Design review of the part built by this model. Coordinates are the model's own, in mm. A direction names the side the tool comes from. Give positions to 0.01 mm unless a question says otherwise; leave off trailing zeros. Order: outer loops, then holes, each group sorted by start corner. A loop starts at its lowest first (then second) coordinate and runs counter-clockwise, first axis right, second up. Notation, with made-up numbers: M 9.25,81 L 47.25,81 A14 ccw 47.25,91 Z; hole C 68,26 d2. An arc over 180 degrees is marked long. Put each result on its own line as item: value. Start each with the question number.
Autodesk Inventor part; units mm, degrees
ref_plane "YZ Plane" through (0, 0, 0) normal (1, 0, 0) x (0, 1, 0)
ref_plane "XZ Plane" through (0, 0, 0) normal (0, 1, 0) x (-1, 0, 0)
ref_plane "XY Plane" through (0, 0, 0) normal (0, 0, 1) x (1, 0, 0)
sketch "Sketch1" plane through (0, 0, 0) normal (0, 0, 1) x (1, 0, 0)
  line L0 (0, 68.5) -> (0, 6.5)
  line L1 (68, 68.5) -> (78, 58.5)
  line L2 (78, 58.5) -> (78, 16.5)
  line L3 (78, 16.5) -> (68, 6.5)
  line L4 (68, 0) -> (68, 6.5)
  line L5 (68, 68.5) -> (68, 75)
  circle A0 centre (71, 57.5) radius 2.75
  circle A1 centre (71, 17.5) radius 2.75
  line L6 (25, 67.5) -> (34, 67.5)
  line L7 (35, 66.5) -> (35, 43.5)
  line L8 (34, 42.5) -> (25, 42.5)
  line L9 (24, 43.5) -> (24, 66.5)
  line L10 (25, 32.5) -> (34, 32.5)
  line L11 (35, 31.5) -> (35, 8.5)
  line L12 (34, 7.5) -> (25, 7.5)
  line L13 (24, 8.5) -> (24, 31.5)
  arc A2 (25, 67.5) -> (24, 66.5) centre (25, 66.5) ccw
  arc A3 (35, 66.5) -> (34, 67.5) centre (34, 66.5) ccw
  arc A4 (34, 42.5) -> (35, 43.5) centre (34, 43.5) ccw
  arc A5 (24, 43.5) -> (25, 42.5) centre (25, 43.5) ccw
  arc A6 (25, 32.5) -> (24, 31.5) centre (25, 31.5) ccw
  arc A7 (24, 8.5) -> (25, 7.5) centre (25, 8.5) ccw
  arc A8 (34, 7.5) -> (35, 8.5) centre (34, 8.5) ccw
  arc A9 (35, 31.5) -> (34, 32.5) centre (34, 31.5) ccw
  line L14 (29.5, 67.5) -> (29.5, 7.5) construction
  circle A10 centre (6, 64.5) radius 5 construction
  circle A11 centre (6, 64.5) radius 2.75
  circle A12 centre (6, 10.5) radius 5 construction
  circle A13 centre (6, 10.5) radius 2.75
  line L15 (0, 64.5) -> (72, 64.5) construction
  line L16 (0, 10.5) -> (72, 10.5) construction
  line L17 (0, 6.5) -> (16, 6.5)
  line L18 (16, 6.5) -> (16, 0)
  line L19 (0, 68.5) -> (16, 68.5)
  line L20 (16, 68.5) -> (16, 75)
  line L21 (46, 75) -> (46, 68.5)
  line L22 (46, 68.5) -> (64, 68.5)
  line L23 (64, 68.5) -> (64, 75)
  line L24 (46, 0) -> (46, 6.5)
  line L25 (46, 6.5) -> (64, 6.5)
  line L26 (64, 6.5) -> (64, 0)
  line L27 (68, 75) -> (64, 75)
  line L28 (46, 75) -> (16, 75)
  line L29 (16, 0) -> (46, 0)
  line L30 (64, 0) -> (68, 0)
  line L31 (8, 60.5) -> (16, 60.5)
  line L32 (16, 60.5) -> (16, 54)
  line L33 (16, 54) -> (8, 54)
  line L34 (8, 54) -> (8, 60.5)
  line L35 (8, 21) -> (16, 21)
  line L36 (16, 21) -> (16, 14.5)
  line L37 (16, 14.5) -> (8, 14.5)
  line L38 (8, 14.5) -> (8, 21)
  line L39 (54, 21) -> (62, 21)
  line L40 (62, 21) -> (62, 14.5)
  line L41 (62, 14.5) -> (54, 14.5)
  line L42 (54, 14.5) -> (54, 21)
  line L43 (54, 60.5) -> (62, 60.5)
  line L44 (62, 60.5) -> (62, 54)
  line L45 (62, 54) -> (54, 54)
  line L46 (54, 54) -> (54, 60.5)
  circle A14 centre (14, 37.5) radius 5 construction
  circle A15 centre (46, 37.5) radius 5 construction
  circle A16 centre (46, 37.5) radius 2.75
  circle A17 centre (14, 37.5) radius 2.75
  point P0 (0, 0)
  point P1 (29.5, 37.5)
  point P2 (0, 37.5)
  dimension "d1" = 45
  dimension "d2" = 10
  dimension "d11" = 5.5
  dimension "d12" = 5.5
  dimension "d13" = 7
  dimension "d14" = 11
  dimension "d15" = 11
  dimension "d18" = 1
  dimension "d19" = 11
  dimension "d20" = 25
  dimension "d21" = 25
  dimension "d24" = 38.5
  dimension "d25" = 5.5
  dimension "d26" = 5.5
  dimension "d27" = 10
  dimension "d28" = 10
  dimension "d32" = 6
  dimension "d34" = 68
  dimension "d35" = 6.5
  dimension "d36" = 6.5
  dimension "d37" = 4
  dimension "d38" = 4
  dimension "d40" = 1
  dimension "d41" = 30
  dimension "d42" = 18
  dimension "d43" = 4
  dimension "d44" = 4
  dimension "d45" = 6.5
  dimension "d46" = 6.5
  dimension "d47" = 8
  dimension "d48" = 8
  dimension "d49" = 4
  dimension "d50" = 4
  dimension "d51" = 8
  dimension "d52" = 6
  dimension "d53" = 10
  dimension "d54" = 5.5
  dimension "d55" = 10
  dimension "d56" = 5.5
  dimension "d57" = 14
  dimension "d58" = 32
  dimension "d67" = 54
extrude "Extrusion1" add sketch "Sketch1" along normal blind 6.5
sketch "Sketch2" plane through (0, 0, 6.5) normal (0, 0, 1) x (1, 0, 0)
  line L0 (46, 6.5) -> (64, 6.5)
  line L1 (46, 13) -> (54, 13)
  line L2 (54, 13) -> (54, 6.5)
  line L3 (54, 6.5) -> (46, 6.5)
  line L4 (46, 6.5) -> (46, 13)
  line L5 (46, 0) -> (46, 6.5)
  point P0 (0, 0)
  dimension "d61" = 6.5
  dimension "d62" = 8
extrude "Extrusion2" cut sketch "Sketch2" against normal through all
properties part number "x_motor_middle" material "Plywood, Finish"
1. To check wall thickness, follow probe 1 along Y at (x, z) = (14, 3); probe 2 along Y at (x, z) = (57, 5.5); probe 3 along Y at (x, z) = (6, 4). State the ranges of each line that lie inside material, in increasing order.
2. Consider section B-B on y = 17.5. Give the boundary of the cut face in (x, z).
3. Consider section D-D on x = 60. Give the boundary of the cut face in (y, z), then the cut area to 4 significant figures.
4. The part is to be moulded in two halves that separate along X. For faces 1 (the flat face through (66, 75, 3)), 2 (the flat face through (16, 72, 3)), 3 (the cylindrical face through (5.642, 61.773, 3.204)), say which applies: +X half, -X half, draft (parallel to the pull), parting line (faces both ways), or undercut.
5. Insertion check: pin 1 (3 mm diameter, centred on x = 11.5, z = 2, fed in from -Y); pin 2 (2 mm diameter, centred on x = 50.5, z = 4, fed in from +Y); pin 3 (3 mm diameter, centred on y = 73.5, z = 2.5, fed in from -X). Each pin has a flat end and moves straight along its axis. Give the tip position at first contact, or say it passes through.
6. Consider section C-C on y = 29.5. Give the boundary of the cut face in (x, z), then the cut area to 4 significant figures.
7. Consider section A-A on x = 6. Give the boundary of the cut face in (y, z), then the cut area to 4 significant figures.
8. Machinability: for faces 4 (the flat face through (62, 57, 3)), 5 (the flat face through (54, 10, 3)), 6 (the flat face through (31, 75, 3)), which of the approach directions +Z, -Z, +X, -X, +Y, -Y give a long, thin tool a straight path to every point of the face, cutting with its end or side? Answer none if there is none.
Returned:
1. probe 1: y = 6.5 to 14.5, 21 to 34.75, 40.25 to 54, 60.5 to 68.5
1. probe 2: y = 6.5 to 14.5, 21 to 54, 60.5 to 68.5
1. probe 3: y = 6.5 to 7.75, 13.25 to 61.75, 67.25 to 68.5
2. outline: M 0,0 L 8,0 L 8,6.5 L 0,6.5 Z; M 16,0 L 24,0 L 24,6.5 L 16,6.5 Z; M 35,0 L 54,0 L 54,6.5 L 35,6.5 Z; M 62,0 L 68.25,0 L 68.25,6.5 L 62,6.5 Z; M 73.75,0 L 78,0 L 78,6.5 L 73.75,6.5 Z
3. outline: M 6.5,0 L 14.5,0 L 14.5,6.5 L 6.5,6.5 Z; M 21,0 L 54,0 L 54,6.5 L 21,6.5 Z; M 60.5,0 L 68.5,0 L 68.5,6.5 L 60.5,6.5 Z
3. area: 318.5 mm2
4. face 1: draft
4. face 2: -X half
4. face 3: undercut
5. pin 1: stops at y = 6.5
5. pin 2: stops at y = 68.5
5. pin 3: stops at x = 16
6. outline: M 0,0 L 24,0 L 24,6.5 L 0,6.5 Z; M 35,0 L 78,0 L 78,6.5 L 35,6.5 Z
6. area: 435.5 mm2
7. outline: M 6.5,0 L 7.75,0 L 7.75,6.5 L 6.5,6.5 Z; M 13.25,0 L 61.75,0 L 61.75,6.5 L 13.25,6.5 Z; M 67.25,0 L 68.5,0 L 68.5,6.5 L 67.25,6.5 Z
7. area: 331.5 mm2
8. face 4: +Z, -Z
8. face 5: +Z, -Z, -Y
8. face 6: +Z, -Z, +X, -X, +Y
